Can you work these out from the model? Positions are in its coordinate system, mm. Coordinates: 2 decimals unless noted, no trailing zeros. Order: outer loops, then holes, each group sorted by start corner. A loop starts at its lowest first (then second) coordinate and runs counter-clockwise, first axis right, second up. Notation, with made-up numbers: M 77.5,43 L 118.5,43 A13 ccw 118.5,67 Z; hole C 52,17 d2. An arc over 180 degrees is marked long. Answer as CSV lines item,"result". Start each with the question number.
1. If we section it at B-B (y = 65.5): List the corners of the cut face in (x, z) for me, plus the area to 3 significant figures.
2. If we section it at A-A (x = -86): List the corners of the cut face in (y, z) for me.
3. If we section it at C-C (z = 0.4): List the corners of the cut face in (x, y) for me.
4. If we section it at D-D (x = -68.5): List the corners of the cut face in (y, z) for me.
5. Will this pin go through, and if not, where does the flat tip stop? pin 1 (0.6 mm diameter, centred on x = -40, z = 1, fed in from +Y).
6. I need wall thicknesses on line 1 along X through (y, z) = (107, 0.3); line 2 along Y through (x, z) = (-52, 0.3); line 3 along Y through (x, z) = (-92.5, 1.4). Which ranges of each line are inside material? Lowest first, please. Write a range as from..to.
```python
from build123d import *

# Parameters (mm, degrees)
EXTRUDE_1_DEPTH     = 2
CUT_EXTRUDE_1_DEPTH = 2


with BuildPart() as part:
    # 草图1 → 凸台-拉伸1 (new body)
    with BuildSketch(Plane.XY):
        Polygon((-83, 62.119161838), (0, 62.119161838), (0, 116.342711697), (32, 116.342711697), (32, 62.119161838), (32, -109.880838162), (-115, -109.880838162), (-115, 62.119161838), (-115, 116.342711697), (-83, 116.342711697), align=None)
    extrude(amount=EXTRUDE_1_DEPTH)

    # 草图2 → 切除-拉伸1 (cut)
    with BuildSketch(Plane.XY.offset(2)):
        with BuildLine():
            Line((-20.227487309, -41.431118444), (4.13099273, -41.431118444))
            ThreePointArc((4.13099273, -41.431118444), (8.13099273, -45.431118444), (4.13099273, -49.431118444))
            Line((4.13099273, -49.431118444), (-20.227487309, -49.431118444))
            ThreePointArc((-20.227487309, -49.431118444), (-24.227487309, -45.431118444), (-20.227487309, -41.431118444))
        make_face()
        with BuildLine():
            Line((-95.572678874, -30.135740054), (-83.83609572, -30.135740054))
            ThreePointArc((-83.83609572, -30.135740054), (-80.83609572, -33.135740054), (-83.83609572, -36.135740054))
            Line((-83.83609572, -36.135740054), (-95.572678874, -36.135740054))
            ThreePointArc((-95.572678874, -36.135740054), (-98.572678874, -33.135740054), (-95.572678874, -30.135740054))
        make_face()
        with BuildLine():
            Line((-52.358181563, -30.135740054), (-40.621598408, -30.135740054))
            ThreePointArc((-40.621598408, -30.135740054), (-37.621598408, -33.135740054), (-40.621598408, -36.135740054))
            Line((-40.621598408, -36.135740054), (-52.358181563, -36.135740054))
            ThreePointArc((-52.358181563, -36.135740054), (-55.358181563, -33.135740054), (-52.358181563, -30.135740054))
        make_face()
    extrude(amount=-CUT_EXTRUDE_1_DEPTH, mode=Mode.SUBTRACT)


solid = part.part
```
Solved:
1,outline,"M -115,0 L -83,0 L -83,2 L -115,2 Z; M 0,0 L 32,0 L 32,2 L 0,2 Z"
1,area,"128 mm²"
2,outline,"M -109.88,0 L -36.14,0 L -36.14,2 L -109.88,2 Z; M -30.14,0 L 116.34,0 L 116.34,2 L -30.14,2 Z"
3,outline,"M -115,-109.88 L 32,-109.88 L 32,116.34 L 0,116.34 L 0,62.12 L -83,62.12 L -83,116.34 L -115,116.34 Z; hole M -95.57,-36.14 L -83.84,-36.14 A3 ccw -83.84,-30.14 L -95.57,-30.14 A3 ccw Z; hole M -52.36,-36.14 L -40.62,-36.14 A3 ccw -40.62,-30.14 L -52.36,-30.14 A3 ccw Z; hole M -20.23,-49.43 L 4.13,-49.43 A4 ccw 4.13,-41.43 L -20.23,-41.43 A4 ccw Z"
4,outline,"M -109.88,0 L 62.12,0 L 62.12,2 L -109.88,2 Z"
5,pin 1,"y = 62.12"
6,line 1,"-115..-83, 0..32"
6,line 2,"-109.88..-36.14, -30.14..62.12"
6,line 3,"-109.88..-36.14, -30.14..116.34"
